from build123d import *

# Parameters (mm, degrees)
SKETCH_1_R          = 20.25
SKETCH_1_R_2        = 20
EXTRUDE_1_DEPTH     = 70
CUT_EXTRUDE_1_DEPTH = 40
CUT_EXTRUDE_2_DEPTH = 262.804787716
FILLET_1_R          = 12
FILLET_2_R          = 2
FILLET_3_R          = 8
FILLET_4_R          = 10
SKETCH_5_W          = 70
SKETCH_5_H          = 300
CUT_EXTRUDE_4_DEPTH = 262.804787716


with BuildPart() as part:
    # 草图1 → 凸台-拉伸1 (new body)
    with BuildSketch(Plane.XY):
        with BuildLine():
            Line((64.741912408, 162.198904983), (-40, 12.611951555))
            Line((-40, 12.611951555), (-40, -100))
            Line((-40, -100), (40, -100))
            Line((40, -100), (40, -12.611951555))
            Line((40, -12.611951555), (130.274075951, 116.312790075))
            ThreePointArc((130.274075951, 116.312790075), (120.451051634, 172.021929301), (64.741912408, 162.198904983))
        make_face()
        Circle(SKETCH_1_R, mode=Mode.SUBTRACT)
        with Locations((97.50799418, 139.255847529)):
            Circle(SKETCH_1_R_2, mode=Mode.SUBTRACT)
        with Locations((60.225525817, 86.01096465)):
            Circle(SKETCH_1_R_2, mode=Mode.SUBTRACT)
    extrude(amount=EXTRUDE_1_DEPTH)

    # 草图2 → 切除-拉伸1 (cut)
    with BuildSketch(Plane.XY):
        Polygon((-9.823024318, 55.709139226), (55.709139226, 9.823024318), (170.424426496, 173.653433175), (104.892262953, 219.539548083), align=None)
    extrude(amount=CUT_EXTRUDE_1_DEPTH, mode=Mode.SUBTRACT)

    # 草图3 → 切除-拉伸2 (cut, through all)
    with BuildSketch(Plane.ZY.offset(40)):
        Polygon((70, -32), (45, -32), (45, -65), (70, -71.454972244), align=None)
    extrude(amount=-CUT_EXTRUDE_2_DEPTH, mode=Mode.SUBTRACT)

    # 圆角1
    fillet_1_edges = [part.edges().sort_by_distance(p)[0] for p in [
        (0, -71.454972244, 70),
    ]]
    fillet(fillet_1_edges, radius=FILLET_1_R)

    # 圆角2
    fillet_2_edges = [part.edges().sort_by_distance(p)[0] for p in [
        (0, -65, 45),
    ]]
    fillet(fillet_2_edges, radius=FILLET_2_R)

    # 圆角3
    fillet_3_edges = [part.edges().sort_by_distance(p)[0] for p in [
        (0, -32, 45),
    ]]
    fillet(fillet_3_edges, radius=FILLET_3_R)

    # 圆角4
    fillet_4_edges = [part.edges().sort_by_distance(p)[0] for p in [
        (22.943057454, 32.766081772, 40),
    ]]
    fillet(fillet_4_edges, radius=FILLET_4_R)

    # 镜向1: part across plane


with BuildPart() as part_1:
    add(part.part)
    add(part.part.mirror(Plane(origin=(97.50799418, 139.255847529, 0), x_dir=(1, 0, 0), z_dir=(0, 0, -1))))

    # 草图5 → 切除-拉伸4 (cut, through all)
    with BuildSketch(Plane.ZY.offset(40)):
        with Locations((35, 50)):
            Rectangle(SKETCH_5_W, SKETCH_5_H)
    extrude(amount=-CUT_EXTRUDE_4_DEPTH, mode=Mode.SUBTRACT)


solid = part_1.part
Source: CAD feature listing. Evaluate the final solid. Frame: model axes, mm. A direction names the side the tool comes from. Give positions to 0.01 mm unless a question says otherwise; leave off trailing zeros. Order: outer loops, then holes, each group sorted by start corner. A loop starts at its lowest first (then second) coordinate and runs counter-clockwise, first axis right, second up. Notation, with made-up numbers: (-6.5, 19.25) -> (17.5, 19.25) arc R24 ccw to (17.5, 52.25) -> close; hole circle Ø3 at (-17.75, -32.5). An arc over 180 degrees is marked (long way). Use a Markdown table: item, result.
1) Section query C-C, the plane z = -16. Return the cut outline in (x, y).
Answer list:
| item | result |
|---|---|
| outline | (-40, -100) -> (40, -100) -> (40, -12.61) -> (55.71, 9.82) -> (-9.82, 55.71) -> (-40, 12.61) -> close; hole circle Ø40.5 at (0, 0) |
2) Ray query, line 1 along Y through (x, z) = (10.5, -48) (3 decimals); line 2 along Z through (x, y) = (122, 125); line 3 along X through (y, z) = (-56, -37). Return the intervals inside material, ascending. Write a range as [from, to].
Answer list:
| item | result |
|---|---|
| line 1 | [-100, -65.775], [-33.755, -17.315], [17.315, 84.733] |
| line 2 | [-70, -40] |
| line 3 | [-40, 40] |
3) Section query A-A, the plane y = 0. Return the cut outline in (x, z), then the cut area to 3 significant figures.
Answer list:
| item | result |
|---|---|
| outline | (-40, -70) -> (-20.25, -70) -> (-20.25, 0) -> (-40, 0) -> close; (20.25, -70) -> (48.83, -70) -> (48.83, 0) -> (20.25, 0) -> close |
| area | 3,380 mm² |
4) Contact query for flat-ended pins moving along their axis: P1, Ø2, axis at x = 114, z = -49, coming from the +Y side; P2, Ø1, axis at x = 15, z = -22, coming from the +Y side; P3, Ø10, axis at x = 49.5, z = -52.5, coming from the -Y side. Output: stop coordinate, or through.
Answer list:
| item | result |
|---|---|
| P1 | y = 176.13 |
| P2 | y = 38.68 |
| P3 | y = -6.19 |
5) Section query B-B, the plane z = -57. Return the cut outline in (x, y), then the cut area to 3 significant figures.
Answer list:
| item | result |
|---|---|
| outline | (-40, -100) -> (40, -100) -> (40, -68.1) -> (-40, -68.1) -> close; (-40, -32) -> (40, -32) -> (40, -12.61) -> (130.27, 116.31) arc R40 ccw to (64.74, 162.2) -> (-40, 12.61) -> close; hole circle Ø40.5 at (0, 0); hole circle Ø40 at (60.23, 86.01); hole circle Ø40 at (97.51, 139.26) |
| area | 17,400 mm² |
6) Mould query, pull axis Y, two halves, no side actions, for faces 1 (the flat face through (40, -57, -35)), 2 (the cylindrical face through (0.56, -73.49, -67.554)), 3 (the cylindrical face through (121.166, 171.51, -54.79)). Classes: +Y half, -Y half, draft (parallel to the pull), parting line (faces both ways), or undercut.
Answer list:
| item | result |
|---|---|
| face 1 | draft |
| face 2 | undercut |
| face 3 | parting line |
7) Reachability of faces 4 (the cylindrical face through (115.983, 131.596, -54.79)), 5 (the flat face through (-1, -32, -62)), 6 (the flat face through (81, 100, -40)) from +Z, -Z, +X, -X, +Y, -Y: full face, straight path, thin tool, end or side. Return the list, or none.
Answer list:
| item | result |
|---|---|
| face 4 | +Z, -Z |
| face 5 | -Z, +X, -X |
| face 6 | +Z, +X, +Y |
8) Section query D-D, the plane x = 107.5. Return the cut outline in (y, z), then the cut area to 3 significant figures.
Answer list:
| item | result |
|---|---|
| outline | (83.79, -70) -> (121.93, -70) -> (121.93, -40) -> (83.79, -40) -> close; (156.58, -70) -> (177.99, -70) -> (177.99, -40) -> (156.58, -40) -> close |
| area | 1,790 mm² |
